```python
from build123d import *

# Parameters (mm, degrees)
SKETCH1_W              = 7.7
SKETCH1_H              = 6.7
BOSS_EXTRUDE1_DEPTH    = 3.95
SKETCH2_W              = 0.4
SKETCH2_H              = 1
BOSS_EXTRUDE2_DEPTH    = 1.8
FILLET1_R              = 0.4
LPATTERN1_COUNT        = 2
LPATTERN1_PITCH        = 2.9
FILLET1_OF_LPATTERN1_R = 0.4
FILLET2_R              = 0.8
CUT_EXTRUDE1_DEPTH     = 2.8
FILLET3_R              = 0.45
FILLET4_R              = 0.7
CUT_EXTRUDE2_DEPTH     = 2.8
MIRROR3_START          = 0.55
MIRROR3_DEPTH          = 2.8
MIRROR3_START_2        = -2.95
MIRROR3_2_OUTLINE_W    = 0.4
MIRROR3_2_OUTLINE_H    = 1.8
MIRROR3_2_DEPTH        = 0.2
MIRROR3_START_3        = -0.05
MIRROR3_3_OUTLINE_W    = 0.4
MIRROR3_3_OUTLINE_H    = 1.8
MIRROR3_3_DEPTH        = 0.2
MIRROR3_START_4        = -3.85
MIRROR3_4_DEPTH        = 0.4
SKETCH5_W              = 5.8
SKETCH5_H              = 5
BOSS_EXTRUDE3_DEPTH    = 0.1


with BuildPart() as part:
    # Sketch1 → Boss-Extrude1 (new body)
    with BuildSketch(Plane(origin=(0, 0, 0), x_dir=(1, 0, 0), z_dir=(0, 1, 0))):
        Rectangle(SKETCH1_W, SKETCH1_H)
    extrude(amount=BOSS_EXTRUDE1_DEPTH)

    # Sketch2 → Boss-Extrude2 (add)
    with BuildSketch(Plane.XZ):
        with Locations((3.65, -2.85)):
            Rectangle(SKETCH2_W, SKETCH2_H)
    boss_extrude2 = extrude(amount=BOSS_EXTRUDE2_DEPTH)

    # Fillet1
    fillet1_edges = [part.edges().sort_by_distance(p)[0] for p in [
        (3.65, -1.8, -2.35),
        (3.65, -1.8, -3.35),
    ]]
    fillet(fillet1_edges, radius=FILLET1_R)

    # LPattern1: Boss-Extrude2 ×2
    with Locations(*[(0, 0, i * LPATTERN1_PITCH) for i in range(1, LPATTERN1_COUNT)]):
        add(boss_extrude2)

    # Fillet1 of LPattern1
    fillet1_of_lpattern1_edges = [part.edges().sort_by_distance(p)[0] for p in [
        (3.65, -1.8, 0.55),
        (3.65, -1.8, -0.45),
    ]]
    fillet(fillet1_of_lpattern1_edges, radius=FILLET1_OF_LPATTERN1_R)

    # Fillet2
    fillet2_edges = [part.edges().sort_by_distance(p)[0] for p in [
        (3.85, 3.95, 0),
        (-3.85, 3.95, 0),
    ]]
    fillet(fillet2_edges, radius=FILLET2_R)

    # Sketch3 → Cut-Extrude1 (cut)
    with BuildSketch(Plane.XY.offset(3.35)):
        Polygon((3.85, 1.36), (3.85, 1.88), (3.45, 1.36), (3.45, 0), (3.85, 0), align=None)
    extrude(amount=-CUT_EXTRUDE1_DEPTH, mode=Mode.SUBTRACT)

    # Fillet3
    fillet3_edges = [part.edges().sort_by_distance(p)[0] for p in [
        (3.45, 0, 1.95),
    ]]
    fillet(fillet3_edges, radius=FILLET3_R)

    # Fillet4
    fillet4_edges = [part.edges().sort_by_distance(p)[0] for p in [
        (3.45, 1.36, 1.95),
        (3.85, 1.88, 1.95),
    ]]
    fillet(fillet4_edges, radius=FILLET4_R)

    # Sketch4 → Cut-Extrude2 (cut)
    with BuildSketch(Plane.XY.offset(3.35)):
        with BuildLine():
            Line((0, 0.4), (0, 3.55))
            Line((0, 3.55), (3.05, 3.55))
            ThreePointArc((3.05, 3.55), (3.332842712, 3.432842712), (3.45, 3.15))
            Line((3.45, 3.15), (3.45, 2.118085363))
            ThreePointArc((3.45, 2.118085363), (3.434021266, 2.021483497), (3.387787197, 1.935172134))
            Line((3.387787197, 1.935172134), (3.278113612, 1.792596474))
            ThreePointArc((3.278113612, 1.792596474), (3.108588692, 1.476121479), (3.05, 1.121914637))
            Line((3.05, 1.121914637), (3.05, 0.85))
            ThreePointArc((3.05, 0.85), (2.918198052, 0.531801948), (2.6, 0.4))
            Line((2.6, 0.4), (0, 0.4))
        make_face()
    extrude(amount=-CUT_EXTRUDE2_DEPTH, mode=Mode.SUBTRACT)

    # Mirror3: read off the stored shape, not the designer's step
    # Mirror3 outline → Mirror3 (cut)
    with BuildSketch(Plane.XY.offset(MIRROR3_START)):
        with BuildLine():
            Line((-3.85, 1.88), (-3.85, 0))
            Line((-3.85, 0), (-3, 0))
            ThreePointArc((-3, 0), (-3.318198052, 0.131801948), (-3.45, 0.45))
            Line((-3.45, 0.45), (-3.45, 1.121914637))
            ThreePointArc((-3.45, 1.121914637), (-3.487283713, 1.347318991), (-3.595163208, 1.54871217))
            Line((-3.595163208, 1.54871217), (-3.85, 1.88))
        make_face()
        with BuildLine():
            ThreePointArc((-3.05, 0.85), (-2.918198052, 0.531801948), (-2.6, 0.4))
            Line((-2.6, 0.4), (0, 0.4))
            Line((0, 0.4), (0, 3.55))
            Line((0, 3.55), (-3.05, 3.55))
            ThreePointArc((-3.05, 3.55), (-3.332842712, 3.432842712), (-3.45, 3.15))
            Line((-3.45, 3.15), (-3.45, 2.118085363))
            ThreePointArc((-3.45, 2.118085363), (-3.434021266, 2.021483497), (-3.387787197, 1.935172134))
            Line((-3.387787197, 1.935172134), (-3.278113612, 1.792596474))
            ThreePointArc((-3.278113612, 1.792596474), (-3.108588692, 1.476121478), (-3.05, 1.121914637))
            Line((-3.05, 1.121914637), (-3.05, 0.85))
        make_face()
    extrude(amount=MIRROR3_DEPTH, mode=Mode.SUBTRACT)

    # Mirror3 2 outline → Mirror3 2 (add)
    with BuildSketch(Plane.XY.offset(MIRROR3_START_2)):
        with Locations((-3.65, -0.9)):
            Rectangle(MIRROR3_2_OUTLINE_W, MIRROR3_2_OUTLINE_H)
    extrude(amount=MIRROR3_2_DEPTH)

    # Mirror3 3 outline → Mirror3 3 (add)
    with BuildSketch(Plane.XY.offset(MIRROR3_START_3)):
        with Locations((-3.65, -0.9)):
            Rectangle(MIRROR3_3_OUTLINE_W, MIRROR3_3_OUTLINE_H)
    extrude(amount=MIRROR3_3_DEPTH)

    # Mirror3 4 outline → Mirror3 4 (add)
    with BuildSketch(Plane.YZ.offset(MIRROR3_START_4)):
        with BuildLine():
            Line((0, -2.75), (0, -2.35))
            Line((0, -2.35), (-1.4, -2.35))
            ThreePointArc((-1.4, -2.35), (-1.682842712, -2.467157288), (-1.8, -2.75))
            Line((-1.8, -2.75), (0, -2.75))
        make_face()
        with BuildLine():
            Line((-1.8, 0.15), (0, 0.15))
            Line((0, 0.15), (0, 0.55))
            Line((0, 0.55), (-1.4, 0.55))
            ThreePointArc((-1.4, 0.55), (-1.682842712, 0.432842712), (-1.8, 0.15))
        make_face()
        with BuildLine():
            Line((-1.4, -0.45), (0, -0.45))
            Line((0, -0.45), (0, -0.05))
            Line((0, -0.05), (-1.8, -0.05))
            ThreePointArc((-1.8, -0.05), (-1.682842712, -0.332842712), (-1.4, -0.45))
        make_face()
        with BuildLine():
            Line((0, -3.35), (0, -2.95))
            Line((0, -2.95), (-1.8, -2.95))
            ThreePointArc((-1.8, -2.95), (-1.682842712, -3.232842712), (-1.4, -3.35))
            Line((-1.4, -3.35), (0, -3.35))
        make_face()
    extrude(amount=MIRROR3_4_DEPTH)

    # Sketch5 → Boss-Extrude3 (add)
    with BuildSketch(Plane(origin=(0, 3.95, 0), x_dir=(1, 0, 0), z_dir=(0, 1, 0))):
        with Locations((0, 0.15)):
            Rectangle(SKETCH5_W, SKETCH5_H)
    extrude(amount=BOSS_EXTRUDE3_DEPTH)


solid = part.part
```
Could you check a few things on this model? Use its own coordinates, in mm. A direction names the side the tool comes from. Give positions to 0.01 mm unless a question says otherwise; leave off trailing zeros. Loops run counter-clockwise (first coordinate to the right, second up) from the corner with the lowest first, then second, coordinate; pieces in that order, holes last. Notation, with made-up numbers: (-6, 50.25) - (3, 50.25) arc R23 ccw to (3, 69.25) - close; hole circle Ø6 at (-21.75, -31). An arc over 180 degrees is marked (long way). Answer in a Markdown table with one row per item. Add a question column.
Q1. If we section it at A-A (y = -0.8): List the corners of the cut face in (x, z) for me.
Q2. We'd pull the mould along X, two halves only. Please class faces 1 (the face through (-3.61, 3.72, -0.05)), 2 (the face through (3.62, 3.71, -0.05)), 3 (the face through (3.45, 2.6, 2)), 4 (the face through (0, 3.95, 3)): +X half, -X half, draft (parallel to the pull), parting line (faces both ways), or undercut.
Q3. Which directions (+Z, -Z, +X, -X, +Y, -Y) give clear straight access to the entire face, cutting with the end or side of a thin tool? Please do faces 5 (the face through (-3.6, 0.3, 0.55)), 6 (the face through (3.45, -1, 0)), 7 (the face through (-3.45, 2.6, 1.9)).
Q4. If we section it at B-B (z = -1.5): List the corners of the cut face in (x, y) for me.
Q5. If we section it at C-C (x = 0): List the corners of the cut face in (y, z) for me.
Q6. Please list where these lines run through material, in increasing order: L1, parallel to Y at x = 2.5, z = 3; L2, parallel to X at y = 2.15, z = 2.25; L3, parallel to Z at x = -3.5, y = -1.1. Write a range as from..to.
Q7. For pin 1 (3.5 mm diameter, centred on x = 1.5, y = 2.5, fed in from +Z); pin 2 (2 mm diameter, centred on x = 0, z = -0.5, fed in from -Y), each with a flat end and sliding along its axis, tell me the tip position at first contact or that it passes through.
The answers:
| question | item | result |
|---|---|---|
| 1 | outline | (-3.85, -3.35) - (-3.45, -3.35) - (-3.45, -2.35) - (-3.85, -2.35) - close; (-3.85, -0.45) - (-3.45, -0.45) - (-3.45, 0.55) - (-3.85, 0.55) - close; (3.45, -3.35) - (3.85, -3.35) - (3.85, -2.35) - (3.45, -2.35) - close; (3.45, -0.45) - (3.85, -0.45) - (3.85, 0.55) - (3.45, 0.55) - close |
| 2 | face 1 | -X half |
| 2 | face 2 | +X half |
| 2 | face 3 | undercut |
| 2 | face 4 | draft |
| 3 | face 5 | +Z, -X, -Y |
| 3 | face 6 | +Z, -Z, -Y |
| 3 | face 7 | +Z |
| 4 | outline | (-3.85, 0) - (3.85, 0) - (3.85, 3.15) arc R0.8 ccw to (3.05, 3.95) - (2.9, 3.95) - (2.9, 4.05) - (-2.9, 4.05) - (-2.9, 3.95) - (-3.05, 3.95) arc R0.8 ccw to (-3.85, 3.15) - close |
| 5 | outline | (0, -3.35) - (3.95, -3.35) - (3.95, -2.65) - (4.05, -2.65) - (4.05, 2.35) - (3.95, 2.35) - (3.95, 3.35) - (3.55, 3.35) - (3.55, 0.55) - (0.4, 0.55) - (0.4, 3.35) - (0, 3.35) - close |
| 6 | L1 | y = 0..0.4, 3.55..3.95 |
| 6 | L2 | x = -3.85..-3.45, 3.45..3.85 |
| 6 | L3 | z = -3.35..-2.35, -0.45..0.55 |
| 7 | pin 1 | stops at z = 3.35 |
| 7 | pin 2 | stops at y = 0 |
